Part model, mm, in its own coordinate system. Round coordinates to 2 decimals unless told otherwise and drop trailing zeros. Loops run counter-clockwise (first coordinate to the right, second up) from the corner with the lowest first, then second, coordinate; pieces in that order, holes last. Notation, with made-up numbers: M 58,52.25 L 111,52.25 A21 cw 111,71.25 Z; hole C 72,-25.75 d9. An arc over 180 degrees is marked long. Write each question's results on one line, items separated by ' | '.
from build123d import *

# Parameters (mm, degrees)
SKETCH1_R           = 3.25
BOSS_EXTRUDE1_DEPTH = 6.5


with BuildPart() as part:
    # Sketch1 → Boss-Extrude1 (new body)
    with BuildSketch(Plane(origin=(0, 0, 0), x_dir=(1, 0, 0), z_dir=(0, 1, 0))):
        with BuildLine():
            Line((0, 19.75), (37, 19.75))
            ThreePointArc((37, 19.75), (56.75, 0), (37, -19.75))
            Line((37, -19.75), (0, -19.75))
            Line((0, -19.75), (-37, -19.75))
            ThreePointArc((-37, -19.75), (-56.75, 0), (-37, 19.75))
            Line((-37, 19.75), (0, 19.75))
        make_face()
        with Locations(Location((-48.75, 0, 0), (0, 0, 90))):
            Circle(SKETCH1_R, mode=Mode.SUBTRACT)
        with Locations(Location((48.75, 0, 0), (0, 0, 90))):
            Circle(SKETCH1_R, mode=Mode.SUBTRACT)
    extrude(amount=BOSS_EXTRUDE1_DEPTH)


solid = part.part
Item 1: Band-saw the part on D-D on z = -6.5. Give the cut face in (x, y).
Filled sheet:
outline: M -55.65,0 L 55.65,0 L 55.65,6.5 L -55.65,6.5 Z
Item 2: Wall check: L1, parallel to X at y = 4.5, z = 0; L2, parallel to X at y = 5.25, z = 2.5; L3, parallel to Z at x = -48.75, y = 2.5. Give the ranges that are in metal, low to high.
Filled sheet:
L1: -56.75 to -52, -45.5 to 45.5, 52 to 56.75 | L2: -56.59 to -50.83, -46.67 to 46.67, 50.83 to 56.59 | L3: -15.87 to -3.25, 3.25 to 15.87
Item 3: Band-saw the part on B-B on y = 2.25. Give the cut face in (x, z), and give its area (3 significant figures).
Filled sheet:
outline: M -37,-19.75 L 37,-19.75 A19.75 ccw 37,19.75 L -37,19.75 A19.75 ccw Z; hole C -48.75,0 d6.5; hole C 48.75,0 d6.5 | area: 4,080 mm^2
Item 4: Band-saw the part on A-A on z = 0. Give the cut face in (x, y).
Filled sheet:
outline: M -56.75,0 L -52,0 L -52,6.5 L -56.75,6.5 Z; M -45.5,0 L 45.5,0 L 45.5,6.5 L -45.5,6.5 Z; M 52,0 L 56.75,0 L 56.75,6.5 L 52,6.5 Z
Item 5: Band-saw the part on C-C on x = 48.75. Give the cut face in (y, z).
Filled sheet:
outline: M 0,-15.87 L 6.5,-15.87 L 6.5,-3.25 L 0,-3.25 Z; M 0,3.25 L 6.5,3.25 L 6.5,15.87 L 0,15.87 Z
Item 6: Drop a flat-ended pin along its axis: P1, Ø1.5, axis at y = 3, z = -6, coming from the +X side. Give the stop position or say it passes through.
Filled sheet:
P1: x = 56.04
